```python
from build123d import *

# Parameters (mm, degrees)
SKETCH1_W                                       = 1500
SKETCH1_H                                       = 415
RAWMATERIAL_DEPTH                               = 12
CSK_FOR_M5_FLAT_HEAD_MACHINE_SCREW1_D           = 5.2
CSK_FOR_M5_FLAT_HEAD_MACHINE_SCREW1_CSINK_D     = 10.4
CSK_FOR_M5_FLAT_HEAD_MACHINE_SCREW1_CSINK_ANGLE = 90
SKETCH5_W                                       = 80
SKETCH5_H                                       = 55
FRAME_SLOTS_DEPTH                               = 779.267466878


with BuildPart() as part:
    # Sketch1 → RawMaterial (new body)
    with BuildSketch(Plane(origin=(0, 0, 0), x_dir=(1, 0, 0), z_dir=(0, 1, 0))):
        Rectangle(SKETCH1_W, SKETCH1_H)
    extrude(amount=RAWMATERIAL_DEPTH)

    # CSK for M5 Flat Head Machine Screw1 (through all)
    with Locations(Plane(origin=(0, 12, 0), x_dir=(-1, 0, 0), z_dir=(0, 1, 0))):
        with Locations((-694, -102.5), (-694, 87.5), (-400, -12.5), (400, -12.5), (694, 87.5), (694, -102.5), (0, -12.5)):
            CounterSinkHole(CSK_FOR_M5_FLAT_HEAD_MACHINE_SCREW1_D / 2, CSK_FOR_M5_FLAT_HEAD_MACHINE_SCREW1_CSINK_D / 2, counter_sink_angle=CSK_FOR_M5_FLAT_HEAD_MACHINE_SCREW1_CSINK_ANGLE)

    # Sketch5 → Frame Slots (cut, through all)
    with BuildSketch(Plane.XZ):
        with Locations((-710, -180)):
            Rectangle(SKETCH5_W, SKETCH5_H)
        with Locations((710, -180)):
            Rectangle(SKETCH5_W, SKETCH5_H)
    extrude(amount=-FRAME_SLOTS_DEPTH, mode=Mode.SUBTRACT)


solid = part.part
```
Model file for the job. Use its own axes, mm. Coordinates: 2 decimals unless noted, no trailing zeros. Order: outer loops, then holes, each group sorted by start corner. A loop starts at its lowest first (then second) coordinate and runs counter-clockwise, first axis right, second up. Notation, with made-up numbers: (-4, 33) - (49, 33) arc R27 cw to (49, 63) - close; hole circle Ø10 at (77, 89.25). An arc over 180 degrees is marked (long way). Return JSON: item names as keys, results as strings. Group by question number.
1) Flat gauge pins, fed straight in: P1, Ø6, axis at x = -694, y = 3.5, coming from the -Z side; P2, Ø7, axis at x = 400, z = -12.5, coming from the +Y side; P3, Ø3, axis at x = -400, z = -12.5, coming from the +Y side; P4, Ø6, axis at y = 4.5, z = -189.5, coming from the -X side. Where does each tip first touch, or does it go through?
2) Saw through at A-A, the plane z = -174.5. Write the cut outline in (x, y), plus the area to 3 significant figures.
3) Probe line 1 (Z direction, x = 694, y = 7.5); line 2 (X direction, y = 5.25, z = -12.5); line 3 (Z direction, x = -400, y = 6). List the from-to ranges inside material, lowest first. Write a range as from..to.
Values found:
{
 "1": {"P1": "stops at z = -152.5", "P2": "stops at y = 10.3", "P3": "passes through", "P4": "stops at x = -670"},
 "2": {"outline": "(-670, 0) - (670, 0) - (670, 12) - (-670, 12) - close", "area": "16,100 mm²"},
 "3": {"line 1": "z = -152.5..-105.1, -99.9..84.9, 90.1..207.5", "line 2": "x = -750..-402.6, -397.4..-2.6, 2.6..397.4, 402.6..750", "line 3": "z = -207.5..-15.1, -9.9..207.5"}
}
